Input: dimensioned drawing with shaded views. Units: mm. Origin: part minimum x, y, z. Give positions to 0.01 mm unless a question says otherwise; leave off trailing zeros. Order: outer loops, then holes, each group sorted by start corner. A loop starts at its lowest first (then second) coordinate and runs counter-clockwise, first axis right, second up.
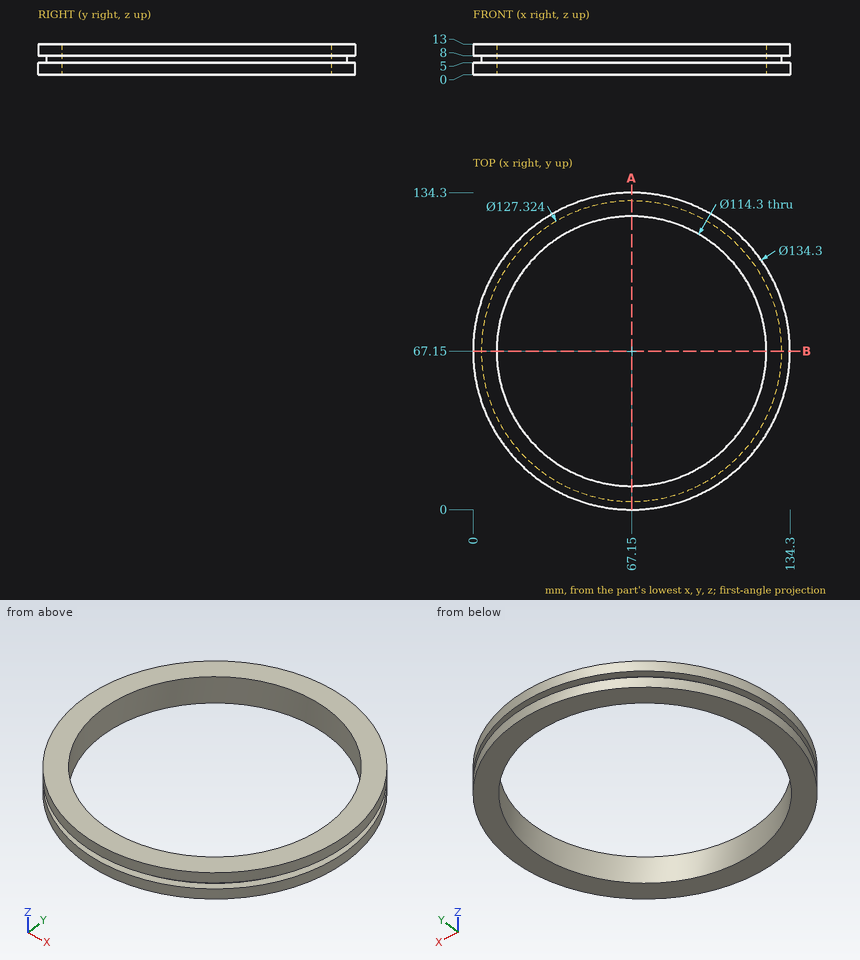
1) Pin query (flat end, axial travel): pin 1 (1 mm diameter, centred on x = 112.5, y = 35.5, fed in from -Z); pin 2 (1.5 mm diameter, centred on y = 73, z = 8.5, fed in from +X); pin 3 (5 mm diameter, centred on y = 24.5, z = 5, fed in from +X); pin 4 (5 mm diameter, centred on y = 111, z = 11.5, fed in from +X). Return the tip coordinate at first contact, or that it passes through.
Report:
pin 1: passes through
pin 2: stops at x = 134.11
pin 3: stops at x = 120.97
pin 4: stops at x = 120.06
2) Section query A-A, the plane x = 67.15. Return the cut outline in (y, z), and give its area (3 significant figures).
Report:
outline: (0, 0) - (10, 0) - (10, 13) - (0, 13) - (0, 8) - (3.49, 8) - (3.49, 5) - (0, 5) - close; (124.3, 0) - (134.3, 0) - (134.3, 5) - (130.81, 5) - (130.81, 8) - (134.3, 8) - (134.3, 13) - (124.3, 13) - close
area: 239 mm2
3) Material intervals for L1, parallel to X at y = 68.5, z = 7; L2, parallel to Y at x = 67.15, z = 6.25; L3, parallel to Y at x = 67.15, z = 10, sorted ascending.
Report:
L1: x = 3.5 to 10.02, 124.28 to 130.8
L2: y = 3.49 to 10, 124.3 to 130.81
L3: y = 0 to 10, 124.3 to 134.3
